```python
from build123d import *

# Parameters (mm, degrees)
BOSS_EXTRUDE1_DEPTH = 30
FILLET10_R          = 2
FILLET11_R          = 2
SKETCH4_W           = 40
SKETCH4_H           = 16.42245212
CUT_EXTRUDE1_DEPTH  = 30
FILLET12_R          = 2


with BuildPart() as part:
    # Sketch2 → Boss-Extrude1 (new body)
    with BuildSketch(Plane.XY):
        Polygon((-70.922010647, 6.21881141), (23.946585559, 6.21881141), (29.020925711, 4.371902636), (28.507895496, 2.962363705), (22.467605346, 5.160849526), (-64.922010647, 5.160849526), (-70.922010647, 6.060990271), align=None)
    extrude(amount=BOSS_EXTRUDE1_DEPTH)

    # Fillet10
    fillet10_edges = [part.edges().sort_by_distance(p)[0] for p in [
        (28.764410604, 3.667133171, 30),
        (28.764410604, 3.667133171, 0),
    ]]
    fillet(fillet10_edges, radius=FILLET10_R)

    # Fillet11
    fillet11_edges = [part.edges().sort_by_distance(p)[0] for p in [
        (23.946585559, 6.21881141, 15),
    ]]
    fillet(fillet11_edges, radius=FILLET11_R)

    # Sketch4 → Cut-Extrude1 (cut)
    with BuildSketch(Plane.XZ.offset(-5.160849526)):
        with Locations((-34.922010647, 5.78877394)):
            Rectangle(SKETCH4_W, SKETCH4_H)
        with BuildLine():
            Line((-59.68856271, 6.67422642), (-59.68856271, 15))
            ThreePointArc((-59.68856271, 15), (-60.922010647, 16.233447938), (-62.155458585, 15))
            Line((-62.155458585, 15), (-62.155458585, 6.67422642))
            ThreePointArc((-62.155458585, 6.67422642), (-60.922010647, 5.440778483), (-59.68856271, 6.67422642))
        make_face()
        with BuildLine():
            Line((-7.739956374, 6.67422642), (-7.739956374, 15))
            ThreePointArc((-7.739956374, 15), (-8.922010647, 16.182054274), (-10.104064921, 15))
            Line((-10.104064921, 15), (-10.104064921, 6.67422642))
            ThreePointArc((-10.104064921, 6.67422642), (-8.922010647, 5.492172147), (-7.739956374, 6.67422642))
        make_face()
    extrude(amount=-CUT_EXTRUDE1_DEPTH, mode=Mode.SUBTRACT)

    # Fillet12
    fillet12_edges = [part.edges().sort_by_distance(p)[0] for p in [
        (-54.922010647, 5.689830468, 0),
        (-14.922010647, 5.689830468, 0),
        (-54.922010647, 5.689830468, 14),
        (-14.922010647, 5.689830468, 14),
    ]]
    fillet(fillet12_edges, radius=FILLET12_R)


solid = part.part
```
The listing builds one solid part. Answer for the finished solid, in the listing's coordinates (mm). A direction names the side the tool comes from. Coordinates: 2 decimals unless noted, no trailing zeros. Loops run counter-clockwise (first coordinate to the right, second up) from the corner with the lowest first, then second, coordinate; pieces in that order, holes last. Notation, with made-up numbers: M 41,20.5 L 81,20.5 A20 cw 81,48.5 Z; hole C 64,-39.5 d10. An arc over 180 degrees is marked long. Answer as CSV lines item,"result". Start each with the question number.
(1) The part is cut by section A-A (z = 4.5). Give the vertices of the cut face in (x, y).
(2) Find the intervals of material crossed by L1, parallel to Y at x = -11.5, z = 6.25, in increasing order. Write a range as [from, to].
(3) The mould has two halves that part along X. Classify faces 1 (the flat face through (-21, 6, 30)), 2 (the flat face through (25.53, 4.046, 14.79)), 3 (the cylindrical face through (-14.32, 5.68, 0.57)): pulls with the +X half, pulls with the -X half, needs draft (parallel to the pull), parting line crosses it, or undercut.
(4) The part is cut by section B-B (z = 8.75). Give the vertices of the cut face in (x, y), and give its area (3 significant figures).
(5) Given pin 1 (1.2 mm diameter, centred on y = 5.5, z = 8.5, fed in from -X); pin 2 (1.2 mm diameter, centred on x = -27, y = 5.5, fed in from -Z); pin 3 (6 mm diameter, centred on x = -10, z = 22.5, fed in from -Y), each flat-ended and moving along its own axis, determine where each tip first touches the part or whether it passes through.
(6) For faces 4 (the cylindrical face through (-15.492, 5.697, 13.399)), 5 (the flat face through (-21, 5.161, 18)), 6 (the flat face through (26.616, 5.247, 14.79)), determine the directions among +Z, -Z, +X, -X, +Y, -Y from which every point of the face is accessible in a straight line to the end or side of a thin tool.
(7) The part is cut by section D-D (x = -48). Give the vertices of the cut face in (y, z).
(8) The part is cut by section C-C (z = 23.5). Give the vertices of the cut face in (x, y).
Determined:
1,outline,"M -70.92,6.06 L -64.92,5.16 L -54.92,5.16 L -54.92,6.22 L -70.92,6.22 Z; M -14.92,5.16 L 22.47,5.16 L 28.51,2.96 L 29.02,4.37 L 24.28,6.1 A2 ccw 23.59,6.22 L -14.92,6.22 Z"
2,L1,"[5.16, 6.22]"
3,face 1,"needs draft"
3,face 2,"pulls with the -X half"
3,face 3,"undercut"
4,outline,"M -70.92,6.06 L -64.92,5.16 L -62.16,5.16 L -62.16,6.22 L -70.92,6.22 Z; M -59.69,5.16 L -54.92,5.16 L -54.92,6.22 L -59.69,6.22 Z; M -14.92,5.16 L -10.1,5.16 L -10.1,6.22 L -14.92,6.22 Z; M -7.74,5.16 L 22.47,5.16 L 28.51,2.96 L 29.02,4.37 L 24.28,6.1 A2 ccw 23.59,6.22 L -7.74,6.22 Z"
4,area,"58.3 mm2"
5,pin 1,"x = -70.92"
5,pin 2,"z = 14"
5,pin 3,"y = 5.16"
6,face 4,"-Z, +Y, -Y"
6,face 5,"+Z, -Z, -X, -Y"
6,face 6,"+Z, -Z, +X, +Y"
7,outline,"M 5.16,14 L 6.22,14 L 6.22,30 L 5.16,30 Z"
8,outline,"M -70.92,6.06 L -64.92,5.16 L 22.47,5.16 L 28.51,2.96 L 29.02,4.37 L 24.28,6.1 A2 ccw 23.59,6.22 L -70.92,6.22 Z"
